from build123d import *

# Parameters (mm, degrees)
SKETCH1_R           = 2.75
BOSS_EXTRUDE1_DEPTH = 2
FILLET1_R           = 1


with BuildPart() as part:
    # Sketch1 → Boss-Extrude1 (new, symmetric)
    with BuildSketch(Plane.XY):
        Polygon((0, 0), (0, 79), (39, 79), (79, 39), (79, 0), align=None)
        with Locations((9.5, 9.5)):
            Circle(SKETCH1_R, mode=Mode.SUBTRACT)
        with Locations((29.5, 9.5)):
            Circle(SKETCH1_R, mode=Mode.SUBTRACT)
        with Locations((49.5, 9.5)):
            Circle(SKETCH1_R, mode=Mode.SUBTRACT)
        with Locations((9.5, 29.5)):
            Circle(SKETCH1_R, mode=Mode.SUBTRACT)
        with Locations((69.5, 9.5)):
            Circle(SKETCH1_R, mode=Mode.SUBTRACT)
        with Locations((69.5, 29.5)):
            Circle(SKETCH1_R, mode=Mode.SUBTRACT)
        with Locations((49.5, 29.5)):
            Circle(SKETCH1_R, mode=Mode.SUBTRACT)
        with Locations((29.5, 29.5)):
            Circle(SKETCH1_R, mode=Mode.SUBTRACT)
        with Locations((29.5, 49.5)):
            Circle(SKETCH1_R, mode=Mode.SUBTRACT)
        with Locations((29.5, 69.5)):
            Circle(SKETCH1_R, mode=Mode.SUBTRACT)
        with BuildLine():
            Line((6.75, 73), (6.75, 49.5))
            ThreePointArc((6.75, 49.5), (9.5, 46.75), (12.25, 49.5))
            Line((12.25, 49.5), (12.25, 73))
            ThreePointArc((12.25, 73), (9.5, 75.75), (6.75, 73))
        make_face(mode=Mode.SUBTRACT)
    extrude(amount=BOSS_EXTRUDE1_DEPTH, both=True)

    # Fillet1
    fillet1_edges = [part.edges().sort_by_distance(p)[0] for p in [
        (59, 59, 2),
        (19.5, 79, 2),
        (0, 39.5, 2),
        (39.5, 0, 2),
        (79, 19.5, 2),
        (0, 0, 0),
        (0, 79, 0),
        (39, 79, 0),
        (79, 39, 0),
        (79, 0, 0),
    ]]
    fillet(fillet1_edges, radius=FILLET1_R)


solid = part.part
The listing builds one solid part. Answer for the finished solid, in the listing's coordinates (mm). A direction names the side the tool comes from. Coordinates: 2 decimals unless noted, no trailing zeros. Order: outer loops, then holes, each group sorted by start corner. A loop starts at its lowest first (then second) coordinate and runs counter-clockwise, first axis right, second up. Notation, with made-up numbers: M -25.5,5.5 L -21.5,5.5 A14 cw -21.5,26.5 Z; hole C 27.25,43 d3. An arc over 180 degrees is marked long. Use CSV: the item, a comma, the result in double quotes.
Q1. A tool of negligible diameter and unlimited length cuts with its end or side. For faces 1 (the flat face through (59, 59, 0)), 2 (the cylindrical face through (9.44, 46.75, 0.03)), from which of +Z, -Z, +X, -X, +Y, -Y can it reach the whole face along a straight path? Write none if from no direction.
Here are the results:
face 1,"+Z, -Z, +X, +Y"
face 2,"+Z, -Z"
Q2. Section A-A (y = 29.5) is taken. Determine the outline of the cut face in (x, z), then the cut area to 3 significant figures.
Here are the results:
outline,"M 0,-2 L 6.75,-2 L 6.75,2 L 1,2 A1 ccw 0,1 Z; M 12.25,-2 L 26.75,-2 L 26.75,2 L 12.25,2 Z; M 32.25,-2 L 46.75,-2 L 46.75,2 L 32.25,2 Z; M 52.25,-2 L 66.75,-2 L 66.75,2 L 52.25,2 Z; M 72.25,-2 L 79,-2 L 79,1 A1 ccw 78,2 L 72.25,2 Z"
area,"228 mm2"
Q3. Straight lines are drawn through the part: L1, parallel to Y at x = 29.5, z = -0.1; L2, parallel to X at y = 10, z = -0.95; L3, parallel to Y at x = 9.5, z = 0.7. For each, find the intervals that lie inside material, in ascending order.
Here are the results:
L1,"0 to 6.75, 12.25 to 26.75, 32.25 to 46.75, 52.25 to 66.75, 72.25 to 79"
L2,"0 to 6.8, 12.2 to 26.8, 32.2 to 46.8, 52.2 to 66.8, 72.2 to 79"
L3,"0 to 6.75, 12.25 to 26.75, 32.25 to 46.75, 75.75 to 79"
Q4. Section B-B (z = -0.25) is taken. Give the number of separate pieces and of enclosed holes in the cut face, then the cut area to 3 significant figures.
Here are the results:
separate pieces,"1"
enclosed holes,"11"
area,"5,050 mm2"
Q5. Determine the mould class of faces 3 (the flat face through (20, 79, 0)), 4 (the flat face through (0, 39, 0)), 5 (the cylindrical face through (27.473, 51.359, -0.028)), 6 (the cylindrical face through (46.753, 9.621, -0.028)) for opening direction X: pulls with the +X half, pulls with the -X half, needs draft (parallel to the pull), parting line crosses it, or undercut.
Here are the results:
face 3,"needs draft"
face 4,"pulls with the -X half"
face 5,"undercut"
face 6,"undercut"
